Verification items for the finished model (mm, model axes). A direction names the side the tool comes from. Give positions to 0.01 mm unless a question says otherwise; leave off trailing zeros. Loops run counter-clockwise (first coordinate to the right, second up) from the corner with the lowest first, then second, coordinate; pieces in that order, holes last. Notation, with made-up numbers: (22.5, -25.5) - (74.5, -25.5) arc R22 ccw to (74.5, 3.5) - close; hole circle Ø5 at (75, 16). An arc over 180 degrees is marked (long way). One line per item, written item: value. Start each with the question number.
1. Sectioned sample at D-D (x = 3.5). Record the cut outline in (y, z) (3 decimals), plus the area to 3 significant figures.
2. Scan lines: L1, parallel to Y at x = -2.25, z = -4; L2, parallel to Z at x = 6, y = 1.75 (3 decimals); L3, parallel to Y at x = 0, z = -4.5. Record each from-to range of solid material in increasing order. Write a range as [from, to].
3. Gauge pin test, flat ends, axial feed: pin 1 (4 mm diameter, centred on x = 4.826, y = 0, fed in from +Z); pin 2 (3 mm diameter, centred on y = -2.5, z = -2, fed in from -X); pin 3 (1.6 mm diameter, centred on x = 5.5, y = 0, fed in from +Z); pin 4 (1 mm diameter, centred on x = -1.5, y = 4, fed in from -Z) (3 decimals). Record the tip position at first contact, or that the pin passes through.
4. Sectioned sample at B-B (x = 0). Record the cut outline in (y, z) (1 decimal), plus the area to 3 significant figures.
5. Access from +Z, -Z, +X, -X, +Y, -Y to the whole of each face (thin tool, end or side, straight path). Record for faces 1 (the flat face through (5, 0, -3.81)), 2 (the flat face through (-2.397, 4.151, -2.191)), 3 (the cylindrical face through (-0.34, 1.55, -6.14)).
6. Mould release check, pull along X, two halves, no side actions. Record for faces 4 (the cylindrical face through (3.556, -0.974, -1.878)), 5 (the flat face through (2, 0, -4.445)), 6 (the cylindrical face through (-2.54, 0.04, -2.19)): pulls with the +X half, pulls with the -X half, needs draft (parallel to the pull), parting line crosses it, or undercut.
7. Sectioned sample at A-A (z = -3). Record the cut outline in (x, y) (1 decimal).
8. Sectioned sample at C-C (y = -0.5). Record the cut outline in (x, z) (3 decimals), plus the area to 3 significant figures.
from build123d import *

# Parameters (mm, degrees)
F0_R     = 1.6002
F1_DEPTH = 4.445
F2_DEPTH = 3.81
F3_R     = 1.5875
F4_DEPTH = 3.429


with BuildPart() as f1:
    # F0 (on Top) → F1 (new body)
    with BuildSketch(Plane.XY):
        with BuildLine():
            ThreePointArc((-3.4925, -6.049187), (3.4925, -6.049187), (6.985, 0))
            ThreePointArc((6.985, 0), (3.4925, 6.049187), (-3.4925, 6.049187))
            Line((-3.4925, 6.049187), (-1.27, 2.199705))
            ThreePointArc((-1.27, 2.199705), (1.27, 2.199705), (2.54, 0))
            ThreePointArc((2.54, 0), (1.27, -2.199705), (-1.27, -2.199705))
            Line((-1.27, -2.199705), (-3.4925, -6.049187))
        make_face()
        with Locations((4.826, 0)):
            Circle(F0_R, mode=Mode.SUBTRACT)
        with BuildLine():
            Line((0, 0), (-1.27, 2.199705))
            ThreePointArc((-1.27, 2.199705), (-2.54, 0), (-1.27, -2.199705))
            Line((-1.27, -2.199705), (0, 0))
        make_face()
        with Locations((4.826, 0)):
            Circle(F0_R)
        with BuildLine():
            ThreePointArc((2.54, 0), (1.27, 2.199705), (-1.27, 2.199705))
            Line((-1.27, 2.199705), (0, 0))
            Line((0, 0), (-1.27, -2.199705))
            ThreePointArc((-1.27, -2.199705), (1.27, -2.199705), (2.54, 0))
        make_face()
    extrude(amount=-F1_DEPTH)

    # F0 (on Top) → F2 (cut)
    with BuildSketch(Plane.XY):
        with Locations((4.826, 0)):
            Circle(F0_R)
    extrude(amount=-F2_DEPTH, mode=Mode.SUBTRACT)

    # F3 (on face) → F4 (join)
    with BuildSketch(Plane(origin=(0, 0, -4.445), x_dir=(1, 0, 0), z_dir=(0, 0, -1))):
        Circle(F3_R)
    extrude(amount=F4_DEPTH)


solid = f1.part
Results are:
1. outline: (-6.045, -4.445) - (6.045, -4.445) - (6.045, 0) - (0.896, 0) - (0.896, -3.81) - (-0.896, -3.81) - (-0.896, 0) - (-6.045, 0) - close
1. area: 46.9 mm^2
2. L1: y = [-6.61, -3.9], [-1.18, 1.18], [3.9, 6.61]
2. L2: z = [-4.445, 0]
2. L3: y = [-1.59, 1.59]
3. pin 1: stops at z = 0
3. pin 2: stops at x = -2.33
3. pin 3: stops at z = -3.81
3. pin 4: stops at z = -4.445
4. outline: (-7, -4.4) - (-1.6, -4.4) - (-1.6, -7.9) - (1.6, -7.9) - (1.6, -4.4) - (7, -4.4) - (7, 0) - (-7, 0) - close
4. area: 73.0 mm^2
5. face 1: +Z
5. face 2: +Z, -Z, -X
5. face 3: -Z
6. face 4: undercut
6. face 5: needs draft
6. face 6: pulls with the -X half
7. outline: (-3.5, -6) arc R7 ccw (long way) to (-3.5, 6) - (-1.3, 2.2) arc R2.5 ccw to (-1.3, -2.2) - close; hole circle Ø3.2 at (4.8, 0)
8. outline: (-2.49, -4.445) - (-1.507, -4.445) - (-1.507, -7.874) - (1.507, -7.874) - (1.507, -4.445) - (6.967, -4.445) - (6.967, 0) - (6.346, 0) - (6.346, -3.81) - (3.306, -3.81) - (3.306, 0) - (-2.49, 0) - close
8. area: 40.8 mm^2
